from build123d import *

# Parameters (mm, degrees)
SKETCH2_W                      = 1.704522774
SKETCH2_H                      = 15
CUT_EXTRUDE1_DEPTH             = 20
CUT_EXTRUDE1_DEPTH_BACK        = 20
M5_CLEARANCE_HOLE1_D           = 5.5
M5_CLEARANCE_HOLE1_DEPTH       = 13
M5_CLEARANCE_HOLE1_CSINK_D     = 5.55
M5_CLEARANCE_HOLE1_CSINK_ANGLE = 90
M5_CLEARANCE_HOLE1_TIP         = 1.652366702


with BuildPart() as part:
    # Sketch1 → Revolve1 (revolve)
    with BuildSketch(Plane.XY):
        Polygon((18, 93), (11, 93), (11, 95), (4, 95), (4, 113), (0, 113), (0, 0), (0, -15), (19, -15), (19, -7), (7, -7), (7, 0), (18, 0), (18, 57), align=None)
    revolve(axis=Axis((0, 113, 0), (0, -1, 0)))

    # Sketch2 → Cut-Extrude1 (cut, two sides)
    with BuildSketch(Plane.XY) as cut_extrude1_sk:
        with Locations((3.852261387, 105.5)):
            Rectangle(SKETCH2_W, SKETCH2_H)
    extrude(amount=CUT_EXTRUDE1_DEPTH, mode=Mode.SUBTRACT)
    extrude(cut_extrude1_sk.sketch, amount=-CUT_EXTRUDE1_DEPTH_BACK, mode=Mode.SUBTRACT)

    # M5 Clearance Hole1
    with Locations(Plane(origin=(0, 93, 0), x_dir=(1, 0, 0), z_dir=(0, 1, 0))):
        with Locations((-9.899494937, 9.899494937), (-9.899494937, -9.899494937), (9.899494937, -9.899494937), (9.899494937, 9.899494937)):
            CounterSinkHole(M5_CLEARANCE_HOLE1_D / 2, M5_CLEARANCE_HOLE1_CSINK_D / 2, depth=M5_CLEARANCE_HOLE1_DEPTH, counter_sink_angle=M5_CLEARANCE_HOLE1_CSINK_ANGLE)
            with Locations((0, 0, -(M5_CLEARANCE_HOLE1_DEPTH + M5_CLEARANCE_HOLE1_TIP / 2))):  # 118° drill point
                Cone(0, M5_CLEARANCE_HOLE1_D / 2, M5_CLEARANCE_HOLE1_TIP, mode=Mode.SUBTRACT)


solid = part.part
Geometry: final body of the model. Coordinates: model frame, mm. A direction names the side the tool comes from. Round coordinates to 2 decimals unless told otherwise and drop trailing zeros. Order: outer loops, then holes, each group sorted by start corner. A loop starts at its lowest first (then second) coordinate and runs counter-clockwise, first axis right, second up.
Q1. Section A-A, the plane z = 0. Output: boundary loops of the cut face in (x, y).
Result sheet:
outline: (-19, -15) - (19, -15) - (19, -7) - (7, -7) - (7, 0) - (18, 0) - (18, 93) - (11, 93) - (11, 95) - (4, 95) - (4, 98) - (3, 98) - (3, 113) - (-4, 113) - (-4, 95) - (-11, 95) - (-11, 93) - (-18, 93) - (-18, 0) - (-7, 0) - (-7, -7) - (-19, -7) - close
Q2. Mould query, pull axis Y, two halves, no side actions, for faces 1 (the face through (-2.38, 94.01, -10.74)), 2 (the face through (0, -7, -8)), 3 (the face through (-10.377, 78.635, -9.92)). Classes: released by +Y, released by -Y, zero draft, split by the parting line, or undercut.
Result sheet:
face 1: zero draft
face 2: undercut
face 3: released by +Y
Q3. Section D-D, the plane x = -16. Output: boundary loops of the cut face in (y, z).
Result sheet:
outline: (-15, -10.25) - (-7, -10.25) - (-7, 10.25) - (-15, 10.25) - close; (0, -8.25) - (93, -8.25) - (93, 8.25) - (0, 8.25) - close
Q4. Section C-C, the plane z = -15. Output: boundary loops of the cut face in (x, y).
Result sheet:
outline: (-11.66, -15) - (11.66, -15) - (11.66, -7) - (-11.66, -7) - close; (-9.95, 0) - (9.95, 0) - (9.95, 93) - (-9.95, 93) - close
Q5. Section B-B, the plane x = 0. Output: boundary loops of the cut face in (y, z).
Result sheet:
outline: (-15, -19) - (-7, -19) - (-7, -7) - (0, -7) - (0, -18) - (93, -18) - (93, -11) - (95, -11) - (95, -4) - (113, -4) - (113, 4) - (95, 4) - (95, 11) - (93, 11) - (93, 18) - (0, 18) - (0, 7) - (-7, 7) - (-7, 19) - (-15, 19) - close
Q6. Pin query (flat end, axial travel): pin 1 (7 mm diameter, centred on x = -9.9, z = -9.9, fed in from +Y); pin 2 (1.5 mm diameter, centred on x = 5.5, y = 78, fed in from +Z); pin 3 (6 mm diameter, centred on y = 105.5, z = 0.5, fed in from +X); pin 4 (6 mm diameter, centred on x = -5, z = -3.5, fed in from +Y). Return the tip coordinate at first contact, or that it passes through.
Result sheet:
pin 1: stops at y = 95
pin 2: stops at z = 17.36
pin 3: stops at x = 3
pin 4: stops at y = 113
Q7. Material intervals for probe 1 along Y at (x, z) = (-10.5, -14); probe 2 along Y at (x, z) = (7.5, -7.5); probe 3 along Y at (x, z) = (-3.5, 6), sorted ascending.
Result sheet:
probe 1: y = -15 to -7, 0 to 93
probe 2: y = -15 to -7, 0 to 95
probe 3: y = -15 to 95
Q8. Access query for faces 4 (the face through (0, 0, -8)), 5 (the face through (12.082, 86.397, 11.573)), 6 (the face through (3, 105, 0)), 7 (the face through (-1, 113, 0)). Directions: +Z, -Z, +X, -X, +Y, -Y. A direction counts if a zero-diameter tool reaches every point of the face in a straight line with its end or side. Return the directions, or none.
Result sheet:
face 4: none
face 5: +Y
face 6: +Z, -Z, +X, +Y
face 7: +Z, -Z, +X, -X, +Y
